Build history of the part. All positions in model axes, mm. A direction names the side the tool comes from. Coordinates: 2 decimals unless noted, no trailing zeros. Loops run counter-clockwise (first coordinate to the right, second up) from the corner with the lowest first, then second, coordinate; pieces in that order, holes last.
Item 1: Drill centre lines: line 1 along Y through (x, z) = (-321, -11.5); line 2 along Y through (x, z) = (-160.5, -11.1); line 3 along Y through (x, z) = (-137, -11.15). Where is each one in solid material? Low to high.
Item 2: Cut at B-B (z = -14.15). Count the separate pieces of the cut face and the enclosed holes in it, and give its area (3 significant figures).
Item 3: Mould opens along Y. For faces 1 (the face through (-269, -20.2, -13)), 2 (the face through (-138, 40, -13)), 3 (the face through (49, -1, -13)) say: released by +Y, released by -Y, zero draft, split by the parting line, or undercut.
Item 4: 3-axis set-ups, long thin cutter, end or side, ignore diameter. For faces 4 (the face through (-97.3, 6, -13)), 5 (the face through (-331, -1, -13)): which of +Z, -Z, +X, -X, +Y, -Y reach the whole face in a straight line?
Item 5: Cut at A-A (x = -262.5). List the corners of the cut face in (y, z).
from build123d import *

# Parameters (mm, degrees)
SKETCH1_W           = 380
SKETCH1_H           = 80
SKETCH1_R           = 2.2
BOSS_EXTRUDE1_DEPTH = 6


with BuildPart() as part:
    # Sketch1 → Boss-Extrude1 (new body)
    with BuildSketch(Plane(origin=(0, 0, -15.5), x_dir=(-1, 0, 0), z_dir=(0, 0, -1))):
        with Locations((141, 0)):
            Rectangle(SKETCH1_W, SKETCH1_H)
        with Locations(Location((-9, -30, 0), (0, 0, 180))):
            Circle(SKETCH1_R, mode=Mode.SUBTRACT)
        with Locations(Location((-9, 30, 0), (0, 0, 180))):
            Circle(SKETCH1_R, mode=Mode.SUBTRACT)
        with Locations(Location((-9, 0, 0), (0, 0, 180))):
            Circle(SKETCH1_R, mode=Mode.SUBTRACT)
        with Locations(Location((-39, -30, 0), (0, 0, 180))):
            Circle(SKETCH1_R, mode=Mode.SUBTRACT)
        with Locations(Location((-39, 30, 0), (0, 0, 180))):
            Circle(SKETCH1_R, mode=Mode.SUBTRACT)
        with Locations(Location((-39, 0, 0), (0, 0, 180))):
            Circle(SKETCH1_R, mode=Mode.SUBTRACT)
        with Locations(Location((291, 30, 0), (0, 0, 180))):
            Circle(SKETCH1_R, mode=Mode.SUBTRACT)
        with Locations(Location((321, -30, 0), (0, 0, 180))):
            Circle(SKETCH1_R, mode=Mode.SUBTRACT)
        with Locations(Location((321, 0, 0), (0, 0, 180))):
            Circle(SKETCH1_R, mode=Mode.SUBTRACT)
        with Locations(Location((33.5, -30, 0), (0, 0, 180))):
            Circle(SKETCH1_R, mode=Mode.SUBTRACT)
        with Locations(Location((65.5, 30, 0), (0, 0, 180))):
            Circle(SKETCH1_R, mode=Mode.SUBTRACT)
        with Locations(Location((99.5, -30, 0), (0, 0, 180))):
            Circle(SKETCH1_R, mode=Mode.SUBTRACT)
        with Locations(Location((115.5, 30, 0), (0, 0, 180))):
            Circle(SKETCH1_R, mode=Mode.SUBTRACT)
        with Locations(Location((160.5, -11.5, 0), (0, 0, 180))):
            Circle(SKETCH1_R, mode=Mode.SUBTRACT)
        with Locations(Location((160.5, 18.5, 0), (0, 0, 180))):
            Circle(SKETCH1_R, mode=Mode.SUBTRACT)
        with Locations(Location((179.5, -11.5, 0), (0, 0, 180))):
            Circle(SKETCH1_R, mode=Mode.SUBTRACT)
        with Locations(Location((179.5, 18.5, 0), (0, 0, 180))):
            Circle(SKETCH1_R, mode=Mode.SUBTRACT)
        with Locations(Location((194.5, 30, 0), (0, 0, 180))):
            Circle(SKETCH1_R, mode=Mode.SUBTRACT)
        with Locations(Location((224.5, 30, 0), (0, 0, 180))):
            Circle(SKETCH1_R, mode=Mode.SUBTRACT)
        with Locations(Location((8, 6, 0), (0, 0, 180))):
            Circle(SKETCH1_R, mode=Mode.SUBTRACT)
        with Locations(Location((20, -30, 0), (0, 0, 180))):
            Circle(SKETCH1_R, mode=Mode.SUBTRACT)
        with Locations(Location((8, -18, 0), (0, 0, 180))):
            Circle(SKETCH1_R, mode=Mode.SUBTRACT)
        with Locations(Location((20, 18, 0), (0, 0, 180))):
            Circle(SKETCH1_R, mode=Mode.SUBTRACT)
        with Locations(Location((8, 30, 0), (0, 0, 180))):
            Circle(SKETCH1_R, mode=Mode.SUBTRACT)
        with Locations(Location((20, -6, 0), (0, 0, 180))):
            Circle(SKETCH1_R, mode=Mode.SUBTRACT)
        with Locations(Location((8, -6, 0), (0, 0, 180))):
            Circle(SKETCH1_R, mode=Mode.SUBTRACT)
        with Locations(Location((20, 6, 0), (0, 0, 180))):
            Circle(SKETCH1_R, mode=Mode.SUBTRACT)
        with Locations(Location((8, 18, 0), (0, 0, 180))):
            Circle(SKETCH1_R, mode=Mode.SUBTRACT)
        with Locations(Location((20, 30, 0), (0, 0, 180))):
            Circle(SKETCH1_R, mode=Mode.SUBTRACT)
        with Locations(Location((8, -30, 0), (0, 0, 180))):
            Circle(SKETCH1_R, mode=Mode.SUBTRACT)
        with Locations(Location((20, -18, 0), (0, 0, 180))):
            Circle(SKETCH1_R, mode=Mode.SUBTRACT)
        with Locations(Location((244.5, -30, 0), (0, 0, 180))):
            Circle(SKETCH1_R, mode=Mode.SUBTRACT)
        with Locations(Location((209.5, 30, 0), (0, 0, 180))):
            Circle(SKETCH1_R, mode=Mode.SUBTRACT)
        with Locations(Location((179.5, 30, 0), (0, 0, 180))):
            Circle(SKETCH1_R, mode=Mode.SUBTRACT)
        with Locations(Location((179.5, 3.5, 0), (0, 0, 180))):
            Circle(SKETCH1_R, mode=Mode.SUBTRACT)
        with Locations(Location((160.5, 30, 0), (0, 0, 180))):
            Circle(SKETCH1_R, mode=Mode.SUBTRACT)
        with Locations(Location((160.5, 3.5, 0), (0, 0, 180))):
            Circle(SKETCH1_R, mode=Mode.SUBTRACT)
        with Locations(Location((130.5, 30, 0), (0, 0, 180))):
            Circle(SKETCH1_R, mode=Mode.SUBTRACT)
        with Locations(Location((145.5, 30, 0), (0, 0, 180))):
            Circle(SKETCH1_R, mode=Mode.SUBTRACT)
        with Locations(Location((80.5, 30, 0), (0, 0, 180))):
            Circle(SKETCH1_R, mode=Mode.SUBTRACT)
        with Locations(Location((50.5, 30, 0), (0, 0, 180))):
            Circle(SKETCH1_R, mode=Mode.SUBTRACT)
        with Locations(Location((321, 30, 0), (0, 0, 180))):
            Circle(SKETCH1_R, mode=Mode.SUBTRACT)
        with Locations(Location((291, 0, 0), (0, 0, 180))):
            Circle(SKETCH1_R, mode=Mode.SUBTRACT)
        with Locations(Location((291, -30, 0), (0, 0, 180))):
            Circle(SKETCH1_R, mode=Mode.SUBTRACT)
        with BuildLine():
            Line((280, 15.8), (258, 15.8))
            ThreePointArc((258, 15.8), (255.8, 18), (258, 20.2))
            Line((258, 20.2), (280, 20.2))
            ThreePointArc((280, 20.2), (282.2, 18), (280, 15.8))
        make_face(mode=Mode.SUBTRACT)
        with BuildLine():
            Line((280, -8.2), (258, -8.2))
            ThreePointArc((258, -8.2), (255.8, -6), (258, -3.8))
            Line((258, -3.8), (280, -3.8))
            ThreePointArc((280, -3.8), (282.2, -6), (280, -8.2))
        make_face(mode=Mode.SUBTRACT)
        with BuildLine():
            Line((280, -32.2), (258, -32.2))
            ThreePointArc((258, -32.2), (255.8, -30), (258, -27.8))
            Line((258, -27.8), (280, -27.8))
            ThreePointArc((280, -27.8), (282.2, -30), (280, -32.2))
        make_face(mode=Mode.SUBTRACT)
        with BuildLine():
            Line((280, -20.2), (258, -20.2))
            ThreePointArc((258, -20.2), (255.8, -18), (258, -15.8))
            Line((258, -15.8), (280, -15.8))
            ThreePointArc((280, -15.8), (282.2, -18), (280, -20.2))
        make_face(mode=Mode.SUBTRACT)
        with BuildLine():
            Line((280, 3.8), (258, 3.8))
            ThreePointArc((258, 3.8), (255.8, 6), (258, 8.2))
            Line((258, 8.2), (280, 8.2))
            ThreePointArc((280, 8.2), (282.2, 6), (280, 3.8))
        make_face(mode=Mode.SUBTRACT)
        with BuildLine():
            Line((280, 27.8), (258, 27.8))
            ThreePointArc((258, 27.8), (255.8, 30), (258, 32.2))
            Line((258, 32.2), (280, 32.2))
            ThreePointArc((280, 32.2), (282.2, 30), (280, 27.8))
        make_face(mode=Mode.SUBTRACT)
        with BuildLine():
            Line((31.3, -16.5), (31.3, 30))
            ThreePointArc((31.3, 30), (33.5, 32.2), (35.7, 30))
            Line((35.7, 30), (35.7, -16.5))
            ThreePointArc((35.7, -16.5), (33.5, -18.7), (31.3, -16.5))
        make_face(mode=Mode.SUBTRACT)
        with BuildLine():
            Line((48.5, -27.8), (82.5, -27.8))
            ThreePointArc((82.5, -27.8), (84.7, -30), (82.5, -32.2))
            Line((82.5, -32.2), (48.5, -32.2))
            ThreePointArc((48.5, -32.2), (46.3, -30), (48.5, -27.8))
        make_face(mode=Mode.SUBTRACT)
        with BuildLine():
            Line((97.3, -16.5), (97.3, 30))
            ThreePointArc((97.3, 30), (99.5, 32.2), (101.7, 30))
            Line((101.7, 30), (101.7, -16.5))
            ThreePointArc((101.7, -16.5), (99.5, -18.7), (97.3, -16.5))
        make_face(mode=Mode.SUBTRACT)
        with BuildLine():
            Line((242.3, -16.5), (242.3, 30))
            ThreePointArc((242.3, 30), (244.5, 32.2), (246.7, 30))
            Line((246.7, 30), (246.7, -16.5))
            ThreePointArc((246.7, -16.5), (244.5, -18.7), (242.3, -16.5))
        make_face(mode=Mode.SUBTRACT)
        with BuildLine():
            Line((229.5, -32.2), (114.5, -32.2))
            ThreePointArc((114.5, -32.2), (112.3, -30), (114.5, -27.8))
            Line((114.5, -27.8), (229.5, -27.8))
            ThreePointArc((229.5, -27.8), (231.7, -30), (229.5, -32.2))
        make_face(mode=Mode.SUBTRACT)
    extrude(amount=-BOSS_EXTRUDE1_DEPTH)


solid = part.part
Filled sheet:
1. line 1: y = -40 to -32.2, -27.8 to -2.2, 2.2 to 27.8, 32.2 to 40
1. line 2: y = -40 to -32.2, -27.8 to -13.7, -9.3 to 1.3, 5.7 to 16.3, 20.7 to 27.8, 32.2 to 40
1. line 3: y = -40 to -32.2, -27.8 to 40
2. separate pieces: 1
2. enclosed holes: 55
2. area: 27,700 mm2
3. face 1: undercut
3. face 2: released by +Y
3. face 3: zero draft
4. face 4: +Z, -Z
4. face 5: +Z, -Z, -X, +Y, -Y
5. outline: (-40, -15.5) - (-32.2, -15.5) - (-32.2, -9.5) - (-40, -9.5) - close; (-27.8, -15.5) - (-20.2, -15.5) - (-20.2, -9.5) - (-27.8, -9.5) - close; (-15.8, -15.5) - (-8.2, -15.5) - (-8.2, -9.5) - (-15.8, -9.5) - close; (-3.8, -15.5) - (3.8, -15.5) - (3.8, -9.5) - (-3.8, -9.5) - close; (8.2, -15.5) - (15.8, -15.5) - (15.8, -9.5) - (8.2, -9.5) - close; (20.2, -15.5) - (27.8, -15.5) - (27.8, -9.5) - (20.2, -9.5) - close; (32.2, -15.5) - (40, -15.5) - (40, -9.5) - (32.2, -9.5) - close
